```python
from build123d import *

# Parameters (mm, degrees)
F1_DEPTH = 10
F3_DEPTH = 90


with BuildPart() as f1:
    # F0 (on Front) → F1 (new body)
    with BuildSketch(Plane.XZ):
        Polygon((475, -360), (-475, 260), (-475, 160), (475, -460), align=None)
    extrude(amount=F1_DEPTH)

    # F2 (on face) → F3 (join)
    with BuildSketch(Plane.XZ.offset(10)):
        Polygon((475, -360), (-475, 260), (-475, 250), (475, -370), align=None)
    extrude(amount=F3_DEPTH)


solid = f1.part
```
Could you check a few things on this model? Use its own coordinates, in mm. A direction names the side the tool comes from. Round coordinates to 2 decimals unless told otherwise and drop trailing zeros. Write each loop counter-clockwise with the first axis right and the second up, starting at its lowest first coordinate (ties: lowest second). Pieces come first, ordered by that corner, then holes. Notation, with made-up numbers: M 83.25,-29.75 L 94.25,-29.75 A6 cw 94.25,-25.75 Z; hole C -14.5,56 d4. An arc over 180 degrees is marked long. Answer in a Markdown table with one row per item. Add a question column.
Q1. Imagine slicing it at A-A (x = 19). Please give me the cut outline in (y, z), then the cut area to 3 significant figures.
Q2. Will these pins go through, and if not, where does the flat tip stop? pin 1 Ø6 at (x, y) = (-48, -53.5) entering from +Z; pin 2 Ø10 at (x, y) = (249.5, -50.5) entering from -Z; pin 3 Ø3 at (x, y) = (-60.5, -72) entering from +Z.
Q3. Imagine slicing it at B-B (y = -59). Please give me the cut outline in (x, z).
Q4. On a 3-axis mill with a long thin cutter (end or side, diameter ignored), from which of +Z, -Z, +X, -X, +Y, -Y can I reach the whole of each face in a straight line? I mean faces 1 (the flat face through (-2, -10, -103)), 2 (the flat face through (-475, -28, 251)). Say none if no direction works.
Q5. If I drill on line 1 (Y direction, x = -158, z = -40); line 2 (Z direction, x = 144.5, y = -78); line 3 (X direction, y = -74, z = 126), over which ranges is the centre line in solid material (lowest first)? Write a range as from..to.
Q6. If we mould it in two halves opening along X, with no side actions, what happens to faces 3 (the flat face through (-2, -100, -54)), 4 (the flat face through (475, -9, -392)), 5 (the flat face through (-6.65, -4.93, -145.66))? For each: +X half, -X half, draft (parallel to the pull), parting line (faces both ways), or undercut.
Q7. Imagine slicing it at C-C (z = 214.5). Please give me the cut outline in (x, y), then the cut area to 3 significant figures.
Values:
| question | item | result |
|---|---|---|
| 1 | outline | M -100,-72.4 L -10,-72.4 L -10,-162.4 L 0,-162.4 L 0,-62.4 L -100,-62.4 Z |
| 1 | area | 1,900 mm^2 |
| 2 | pin 1 | z = -16.72 |
| 2 | pin 2 | z = -226.09 |
| 2 | pin 3 | z = -9.54 |
| 3 | outline | M -475,250 L 475,-370 L 475,-360 L -475,260 Z |
| 4 | face 1 | -Z, -X, -Y |
| 4 | face 2 | +Z, -Z, -X, +Y, -Y |
| 5 | line 1 | -10..0 |
| 5 | line 2 | -154.31..-144.31 |
| 5 | line 3 | -285..-269.68 |
| 6 | face 3 | draft |
| 6 | face 4 | +X half |
| 6 | face 5 | -X half |
| 7 | outline | M -475,-10 L -420.6,-10 L -420.6,-100 L -405.28,-100 L -405.28,0 L -475,0 Z |
| 7 | area | 2,080 mm^2 |
